Read the model definition and answer for the solid it produces. Units are mm, in the model's axes. Coordinates: 2 decimals unless noted, no trailing zeros. Loops run counter-clockwise (first coordinate to the right, second up) from the corner with the lowest first, then second, coordinate; pieces in that order, holes last. Notation, with made-up numbers: M -2,10.5 L 19,10.5 A34 cw 19,41.5 Z; hole C -36.5,6.5 d5. An arc over 180 degrees is marked long. Use one line per item in the form item = value. Start each with the question number.
1. The part is cut by section C-C (z = -93). Give the vertices of the cut face in (x, y).
2. The part is cut by section D-D (y = 0.35). Give the number of separate pieces and of enclosed holes in the cut face, plus the area to 3 significant figures.
3. Find the intervals of material crossed by probe 1 along X at (y, z) = (1.3, -93); probe 2 along X at (y, z) = (1.5, -12); probe 3 along X at (y, z) = (1.1, -111), in increasing order. Write a range as [from, to].
4. Flat-ended cylindrical pins translate along their axes: pin 1 (12 mm diameter, centred on x = -95.5, z = -99.5, fed in from -Y); pin 2 (0.6 mm diameter, centred on y = 0.5, z = -72.5, fed in from +X); pin 3 (1 mm diameter, centred on y = 1, z = 1, fed in from -X); pin 4 (1 mm diameter, centred on y = 1, z = 1, fed in from +X). Find the tip coordinate at first contact, or state that the pin passes through.
5. The part is cut by section B-B (z = -25.5). Give the vertices of the cut face in (x, y), plus the area to 3 significant figures.
6. The part is cut by section A-A (x = -70.25). Give the vertices of the cut face in (y, z).
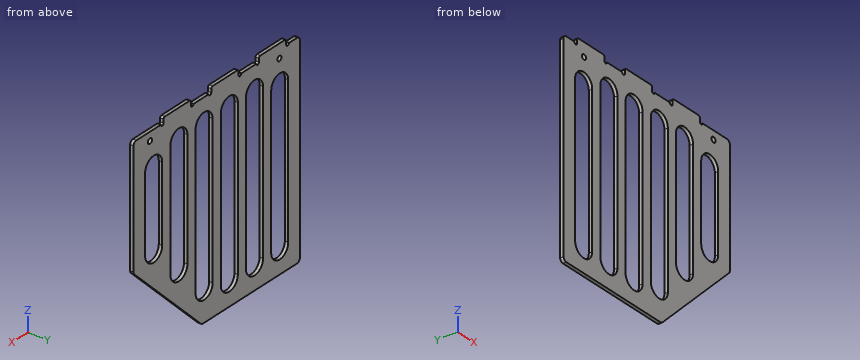
from build123d import *

# Parameters (mm, degrees)
SKETCH_1_R          = 1.5
EXTRUDE_1_DEPTH     = 2
SKETCH_2_R          = 1
CUT_EXTRUDE_1_DEPTH = 172.137371722
CUT_EXTRUDE_2_DEPTH = 172.137371722
FILLET_1_R          = 2
FILLET_2_R          = 1


with BuildPart() as part:
    # 草图1 → 凸台-拉伸1 (new body)
    with BuildSketch(Plane(origin=(0, 0, 0), x_dir=(1, 0, 0), z_dir=(0, 1, 0))):
        Polygon((0, 0), (0, 70), (-50, 120), (-122, 120), (-122, 0), (-112, 0), (-112, -3), (-92, -3), (-92, 0), (-77, 0), (-77, -3), (-57, -3), (-57, 0), (-42, 0), (-42, -3), (-22, -3), (-22, 0), align=None)
        with Locations(Location((-12, 5, 0), (0, 0, 270))):
            Circle(SKETCH_1_R, mode=Mode.SUBTRACT)
        with Locations(Location((-107, 5, 0), (0, 0, 270))):
            Circle(SKETCH_1_R, mode=Mode.SUBTRACT)
    extrude(amount=EXTRUDE_1_DEPTH)

    # 草图2 → 切除-拉伸1 (cut, through all)
    with BuildSketch(Plane(origin=(0, 2, 0), x_dir=(1, 0, 0), z_dir=(0, 1, 0))):
        with Locations((-113, 0)):
            Circle(SKETCH_2_R)
        with Locations((-91, 0)):
            Circle(SKETCH_2_R)
        with Locations((-78, 0)):
            Circle(SKETCH_2_R)
        with Locations((-56, 0)):
            Circle(SKETCH_2_R)
        with Locations((-43, 0)):
            Circle(SKETCH_2_R)
        with Locations((-21, 0)):
            Circle(SKETCH_2_R)
    extrude(amount=-CUT_EXTRUDE_1_DEPTH, mode=Mode.SUBTRACT)

    # 草图3 → 切除-拉伸2 (cut, through all)
    with BuildSketch(Plane(origin=(0, 2, 0), x_dir=(1, 0, 0), z_dir=(0, 1, 0))):
        with BuildLine():
            Line((-101, 105.75), (-101, 19.25))
            ThreePointArc((-101, 19.25), (-107.25, 13), (-113.5, 19.25))
            Line((-113.5, 19.25), (-113.5, 105.75))
            ThreePointArc((-113.5, 105.75), (-107.25, 112), (-101, 105.75))
        make_face()
        with BuildLine():
            Line((-82.5, 105.75), (-82.5, 14.25))
            ThreePointArc((-82.5, 14.25), (-88.75, 8), (-95, 14.25))
            Line((-95, 14.25), (-95, 105.75))
            ThreePointArc((-95, 105.75), (-88.75, 112), (-82.5, 105.75))
        make_face()
        with BuildLine():
            Line((-64, 105.75), (-64, 14.25))
            ThreePointArc((-64, 14.25), (-70.25, 8), (-76.5, 14.25))
            Line((-76.5, 14.25), (-76.5, 105.75))
            ThreePointArc((-76.5, 105.75), (-70.25, 112), (-64, 105.75))
        make_face()
        with BuildLine():
            Line((-45.5, 101.597456736), (-45.5, 14.25))
            ThreePointArc((-45.5, 14.25), (-51.75, 8), (-58, 14.25))
            Line((-58, 14.25), (-58, 101.597456736))
            ThreePointArc((-58, 101.597456736), (-51.75, 107.847456736), (-45.5, 101.597456736))
        make_face()
        with BuildLine():
            Line((-27, 83.097456736), (-27, 14.25))
            ThreePointArc((-27, 14.25), (-33.25, 8), (-39.5, 14.25))
            Line((-39.5, 14.25), (-39.5, 83.097456736))
            ThreePointArc((-39.5, 83.097456736), (-33.25, 89.347456736), (-27, 83.097456736))
        make_face()
        with BuildLine():
            Line((-8.5, 64.597456736), (-8.5, 20.25))
            ThreePointArc((-8.5, 20.25), (-14.75, 14), (-21, 20.25))
            Line((-21, 20.25), (-21, 64.597456736))
            ThreePointArc((-21, 64.597456736), (-14.75, 70.847456736), (-8.5, 64.597456736))
        make_face()
    extrude(amount=-CUT_EXTRUDE_2_DEPTH, mode=Mode.SUBTRACT)

    # 圆角1
    fillet_1_edges = [part.edges().sort_by_distance(p)[0] for p in [
        (-122, 1, 0),
        (-122, 1, -120),
        (-50, 1, -120),
        (0, 1, -70),
        (0, 1, 0),
    ]]
    fillet(fillet_1_edges, radius=FILLET_1_R)

    # 圆角2
    fillet_2_edges = [part.edges().sort_by_distance(p)[0] for p in [
        (-22, 1, 3),
        (-42, 1, 3),
        (-57, 1, 3),
        (-77, 1, 3),
        (-92, 1, 3),
        (-112, 1, 3),
    ]]
    fillet(fillet_2_edges, radius=FILLET_2_R)


solid = part.part
Computed values:
q1.outline = M -122,0 L -113.5,0 L -113.5,2 L -122,2 Z; M -101,0 L -95,0 L -95,2 L -101,2 Z; M -82.5,0 L -76.5,0 L -76.5,2 L -82.5,2 Z; M -64,0 L -58,0 L -58,2 L -64,2 Z; M -45.5,0 L -23,0 L -23,2 L -45.5,2 Z
q2.separate_pieces = 1
q2.enclosed_holes = 8
q2.area = 6,930 mm²
q3.probe_1 = [-122, -113.5], [-101, -95], [-82.5, -76.5], [-64, -58], [-45.5, -23]
q3.probe_2 = [-122, -94.58], [-82.92, -76.08], [-64.42, -57.58], [-45.92, -39.08], [-27.42, 0]
q3.probe_3 = [-122, -110.64], [-103.86, -92.14], [-85.36, -73.64], [-66.86, -41]
q4.pin_1 = 0
q4.pin_2 = -2.2
q4.pin_3 = -112
q4.pin_4 = -22
q5.outline = M -122,0 L -113.5,0 L -113.5,2 L -122,2 Z; M -101,0 L -95,0 L -95,2 L -101,2 Z; M -82.5,0 L -76.5,0 L -76.5,2 L -82.5,2 Z; M -64,0 L -58,0 L -58,2 L -64,2 Z; M -45.5,0 L -39.5,0 L -39.5,2 L -45.5,2 Z; M -27,0 L -21,0 L -21,2 L -27,2 Z; M -8.5,0 L 0,0 L 0,2 L -8.5,2 Z
q5.area = 94.0 mm²
q6.outline = M 0,-120 L 2,-120 L 2,-112 L 0,-112 Z; M 0,-8 L 2,-8 L 2,3 L 0,3 Z
